Design review of the part shown in the three views and the two pictorial views. Dimensions are in mm from the part's minimum x, y and z. A direction names the side the tool comes from. Round coordinates to 2 decimals unless told otherwise and drop trailing zeros. Order: outer loops, then holes, each group sorted by start corner. A loop starts at its lowest first (then second) coordinate and runs counter-clockwise, first axis right, second up.
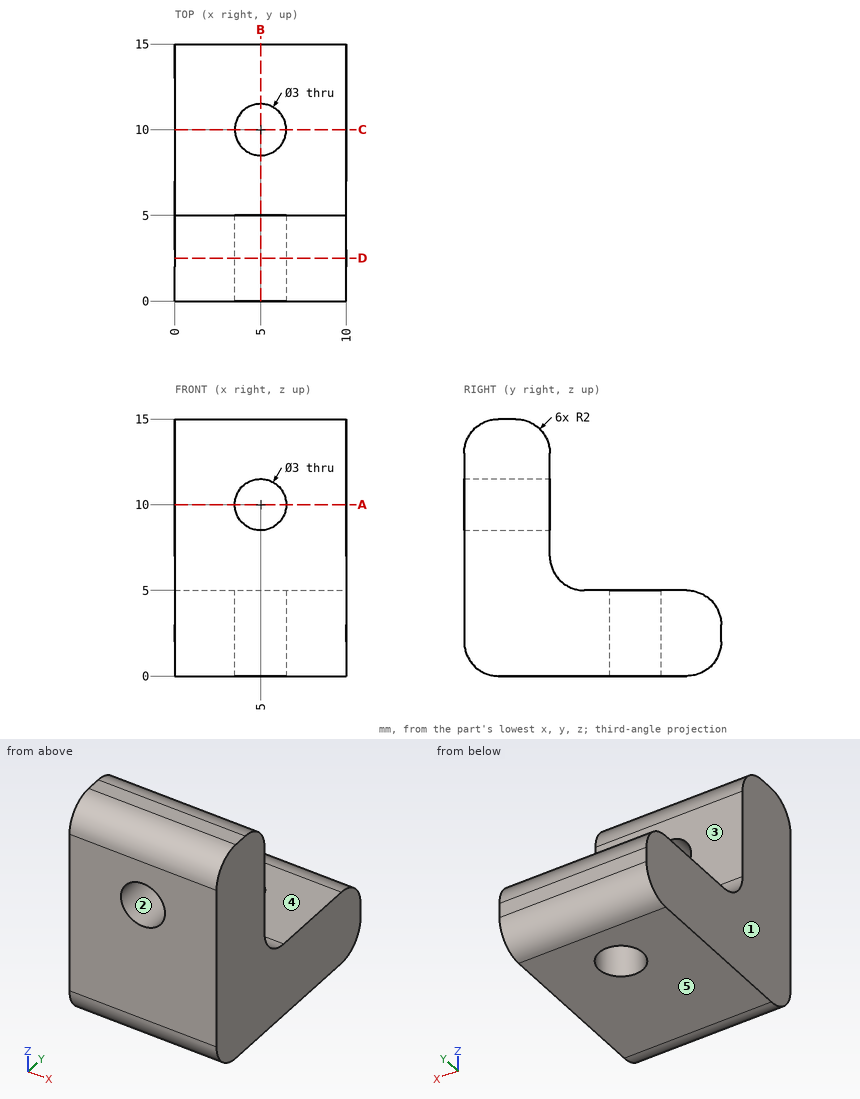
1) Take a section at B-B on x = 5. Give the boundary of the cut face in (y, z).
Results:
outline: (0, 2) arc R2 ccw to (2, 0) - (8.5, 0) - (8.5, 5) - (7, 5) arc R2 cw to (5, 7) - (5, 8.5) - (0, 8.5) - close; (0, 11.5) - (5, 11.5) - (5, 13) arc R2 ccw to (3, 15) - (2, 15) arc R2 ccw to (0, 13) - close; (11.5, 0) - (13, 0) arc R2 ccw to (15, 2) - (15, 3) arc R2 ccw to (13, 5) - (11.5, 5) - close
2) The part is to be moulded in two halves that separate along X. For the marked faces 1, 2 and 3, say which applies: released by +X, released by -X, zero draft, split by the parting line, or undercut.
Results:
face 1: released by -X
face 2: undercut
face 3: zero draft
3) Take a section at D-D on y = 2.5. Give the boundary of the cut face in (x, z).
Results:
outline: (0, 0) - (10, 0) - (10, 15) - (0, 15) - close; hole circle Ø3 at (5, 10)
4) For the marked faces 4 and 5, list the 3-axis set-ups (+Z, -Z, +X, -X, +Y, -Y) from which the entire face can be reached by the end or side of a thin tool; tool diameter is ignored.
Results:
face 4: +Z, +X, -X, +Y
face 5: -Z, +X, -X, +Y, -Y
5) To check wall thickness, follow line 1 along X through (y, z) = (3.7, 10); line 2 along Y through (x, z) = (5, 2.95); line 3 along Z through (x, y) = (3.5, 13). State the ranges of each line that lie inside material, in increasing order.
Results:
line 1: x = 0 to 3.5, 6.5 to 10
line 2: y = 0 to 8.5, 11.5 to 15
line 3: z = 0 to 5
6) Clearance check with flat-ended pins moving along their axes: P1, Ø4, axis at x = 6, z = 4.5, coming from the +Y side; P2, Ø5, axis at x = 2.5, z = 8.5, coming from the +Y side; P3, Ø1.8, axis at x = 5.5, y = 9, coming from the +Z side; P4, Ø5, axis at y = 8, z = 12, coming from the +X side. State where each tip first meets the part, or that it passes through.
Results:
P1: stops at y = 15
P2: stops at y = 5.27
P3: stops at z = 5
P4: passes through
7) Take a section at A-A on z = 10. Give the boundary of the cut face in (x, y), plus the area to 3 significant figures.
Results:
outline: (0, 0) - (3.5, 0) - (3.5, 5) - (0, 5) - close; (6.5, 0) - (10, 0) - (10, 5) - (6.5, 5) - close
area: 35.0 mm2
